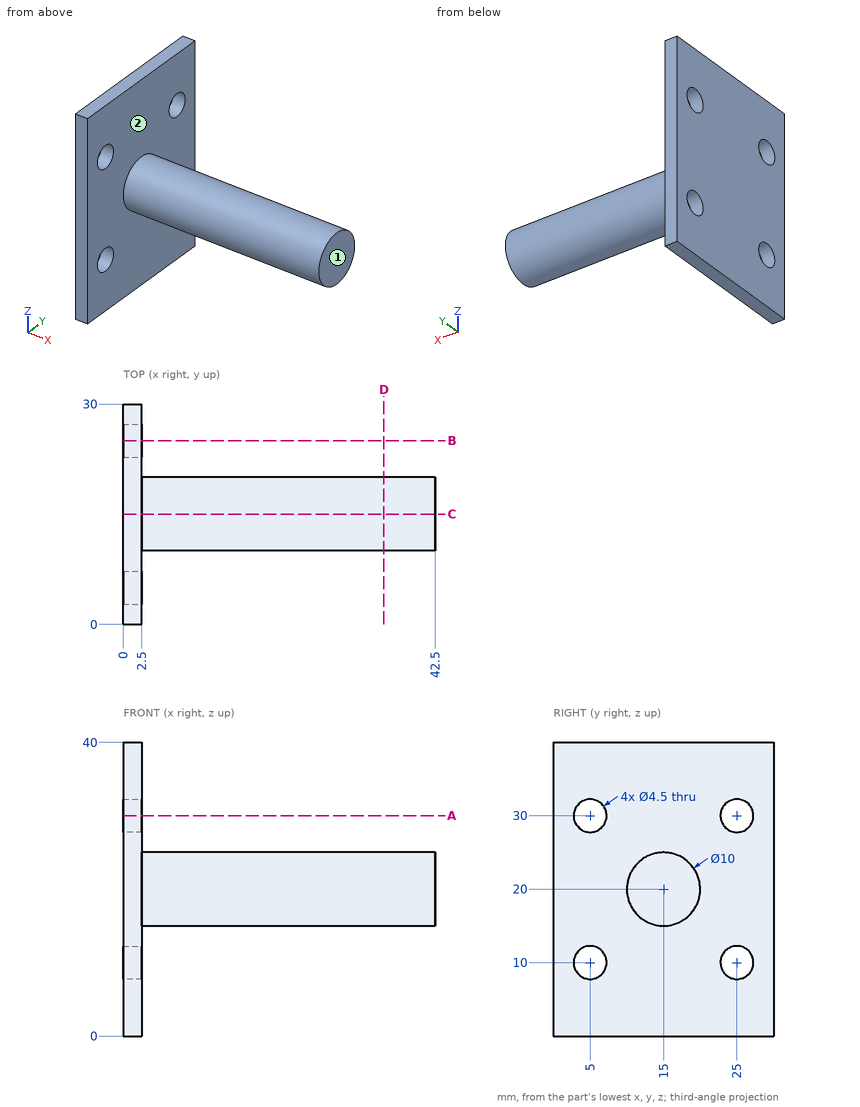
Verification items for this drawing (mm, ordinates from the low corner). A direction names the side the tool comes from. Give positions to 0.01 mm unless a question says otherwise; leave off trailing zeros. Loops run counter-clockwise (first coordinate to the right, second up) from the corner with the lowest first, then second, coordinate; pieces in that order, holes last. Notation, with made-up numbers: M 73,-10 L 108,-10 A10 ccw 108,-4 Z; hole C -31,45.25 d8. An arc over 180 degrees is marked long. Write item = value, one per line. Start each with the question number.
1. Section check A-A, the plane z = 30. Enter the section's corners in (x, y).
2. Section check C-C, the plane y = 15. Enter the section's corners in (x, z), plus the area to 3 significant figures.
3. Thickness scan on probe 1 along Y at (x, z) = (0.5, 30); probe 2 along X at (y, z) = (14.5, 9); probe 3 along Y at (x, z) = (9, 19). Record the ranges inside material, lowest first.
4. Section check B-B, the plane y = 25. Enter the section's corners in (x, z).
5. Tool access check on the marked faces 1 and 2. Record the directions out of +Z, -Z, +X, -X, +Y, -Y that give a thin tool (end or side, any length) a straight path to the whole face; none if there is none.
6. Go/stop test with flat-tipped pins: P1, Ø3, axis at y = 9.5, z = 13.5, coming from the -X side; P2, Ø2, axis at x = 23, y = 13.5, coming from the +Z side; P3, Ø6, axis at y = 5, z = 10, coming from the +X side; P4, Ø3, axis at x = 7, z = 18, coming from the -Y side. Record where each tip stops, or that it passes through.
7. Section check D-D, the plane x = 35.5. Enter the section's corners in (y, z), plus the area to 3 significant figures.
Values follow:
q1.outline = M 0,0 L 2.5,0 L 2.5,2.75 L 0,2.75 Z; M 0,7.25 L 2.5,7.25 L 2.5,22.75 L 0,22.75 Z; M 0,27.25 L 2.5,27.25 L 2.5,30 L 0,30 Z
q2.outline = M 0,0 L 2.5,0 L 2.5,15 L 42.5,15 L 42.5,25 L 2.5,25 L 2.5,40 L 0,40 Z
q2.area = 500 mm^2
q3.probe_1 = 0 to 2.75, 7.25 to 22.75, 27.25 to 30
q3.probe_2 = 0 to 2.5
q3.probe_3 = 10.1 to 19.9
q4.outline = M 0,0 L 2.5,0 L 2.5,7.75 L 0,7.75 Z; M 0,12.25 L 2.5,12.25 L 2.5,27.75 L 0,27.75 Z; M 0,32.25 L 2.5,32.25 L 2.5,40 L 0,40 Z
q5.face_1 = +Z, -Z, +X, +Y, -Y
q5.face_2 = +X
q6.P1 = 0
q6.P2 = 24.97
q6.P3 = 2.5
q6.P4 = 10.03
q7.outline = C 15,20 d10
q7.area = 78.5 mm^2
